```python
from build123d import *

# Parameters (mm, degrees)
SKETCH_1_W                    = 96
SKETCH_1_H                    = 47
EXTRUDE_1_DEPTH               = 6
FILLET_1_R                    = 1
HOLE_WIZARD_M10_1_D           = 8.5
HOLE_WIZARD_M10_1_CSINK_D     = 10.05
HOLE_WIZARD_M10_1_CSINK_ANGLE = 90
SKETCH_2_R                    = 3.3
CUT_EXTRUDE_1_DEPTH           = 10
FILLET_2_R                    = 0.5


with BuildPart() as part:
    # 草图1 → 凸台-拉伸1 (new body)
    with BuildSketch(Plane.XY):
        with Locations((48, -23.5)):
            Rectangle(SKETCH_1_W, SKETCH_1_H)
    extrude(amount=EXTRUDE_1_DEPTH)

    # 圆角1
    fillet_1_edges = [part.edges().sort_by_distance(p)[0] for p in [
        (0, 0, 3),
        (96, 0, 3),
        (96, -47, 3),
        (0, -47, 3),
    ]]
    fillet(fillet_1_edges, radius=FILLET_1_R)

    # M10 螺纹孔1 (through all)
    with Locations(Plane.XY.offset(6)):
        with Locations((28, -23.5), (48, -23.5), (68, -23.5)):
            CounterSinkHole(HOLE_WIZARD_M10_1_D / 2, HOLE_WIZARD_M10_1_CSINK_D / 2, counter_sink_angle=HOLE_WIZARD_M10_1_CSINK_ANGLE)

    # 草图2 → 切除-拉伸1 (cut)
    with BuildSketch(Plane.XY.offset(6)):
        with Locations((83, -6)):
            Circle(SKETCH_2_R)
        with Locations((83, -41)):
            Circle(SKETCH_2_R)
        with Locations((13, -41)):
            Circle(SKETCH_2_R)
        with Locations(Location((13, -6, 0), (0, 0, 180))):
            Circle(SKETCH_2_R)
    extrude(amount=-CUT_EXTRUDE_1_DEPTH, mode=Mode.SUBTRACT)

    # 圆角2
    fillet_2_edges = [part.edges().sort_by_distance(p)[0] for p in [
        (16.3, -6, 6),
        (9.7, -41, 6),
        (79.7, -41, 6),
        (79.7, -6, 6),
    ]]
    fillet(fillet_2_edges, radius=FILLET_2_R)


solid = part.part
```
The model under review builds one solid part; all positions refer to its coordinate system, in mm. Round coordinates to 2 decimals unless told otherwise and drop trailing zeros. Write each loop counter-clockwise with the first axis right and the second up, starting at its lowest first coordinate (ties: lowest second). Pieces come first, ordered by that corner, then holes. Notation, with made-up numbers: (34.25, -36.5) -> (38.25, -36.5) arc R20 ccw to (38.25, -30.5) -> close; hole circle Ø2 at (26, 22). An arc over 180 degrees is marked (long way). Use CSV: the item, a comma, the result in double quotes.
Q1. Consider section A-A (x = 13). Give the boundary of the cut face in (y, z).
Checks:
outline,"(-47, 0) -> (-44.3, 0) -> (-44.3, 5.5) arc R0.5 ccw to (-44.8, 6) -> (-47, 6) -> close; (-37.7, 0) -> (-9.3, 0) -> (-9.3, 5.5) arc R0.5 ccw to (-9.8, 6) -> (-37.2, 6) arc R0.5 ccw to (-37.7, 5.5) -> close; (-2.7, 0) -> (0, 0) -> (0, 6) -> (-2.2, 6) arc R0.5 ccw to (-2.7, 5.5) -> close"
Q2. Mouldability with a two-part tool opening along X and no side actions: class faces 1 (the flat face through (47, -18, 0)), 2 (the cylindrical face through (52.246, -23.313, 2.576)), 3 (the cylindrical face through (64.074, -25.128, 2.576)), 4 (the flat face through (0, -24, 3)) as released by +X, released by -X, zero draft, split by the parting line, or undercut.
Checks:
face 1,"zero draft"
face 2,"undercut"
face 3,"undercut"
face 4,"released by -X"
Q3. For pin 1 Ø7.5 at (x, y) = (83, -6) entering from -Z; pin 2 Ø10 at (x, y) = (68, -23.5) entering from +Z (3 decimals), all flat-tipped, find the tip position at first contact; note any pin that passes through.
Checks:
pin 1,"z = 0"
pin 2,"z = 5.975"
Q4. Consider section B-B (y = -6). Give the boundary of the cut face in (x, z).
Checks:
outline,"(0, 0) -> (9.7, 0) -> (9.7, 5.5) arc R0.5 ccw to (9.2, 6) -> (0, 6) -> close; (16.3, 0) -> (79.7, 0) -> (79.7, 5.5) arc R0.5 ccw to (79.2, 6) -> (16.8, 6) arc R0.5 ccw to (16.3, 5.5) -> close; (86.3, 0) -> (96, 0) -> (96, 6) -> (86.8, 6) arc R0.5 ccw to (86.3, 5.5) -> close"
Q5. To check wall thickness, follow probe 1 along X at (y, z) = (-23.5, 3.85); probe 2 along Y at (x, z) = (82, 2.5); probe 3 along Y at (x, z) = (28, 3.5). State the ranges of each line that lie inside material, in increasing order. Write a range as [from, to].
Checks:
probe 1,"[0, 23.75], [32.25, 43.75], [52.25, 63.75], [72.25, 96]"
probe 2,"[-47, -44.14], [-37.86, -9.14], [-2.86, 0]"
probe 3,"[-47, -27.75], [-19.25, 0]"
Q6. Consider section C-C (z = 2.5). Give the boundary of the cut face in (x, y), then the cut area to 3 significant figures.
Checks:
outline,"(0, -46) arc R1 ccw to (1, -47) -> (95, -47) arc R1 ccw to (96, -46) -> (96, -1) arc R1 ccw to (95, 0) -> (1, 0) arc R1 ccw to (0, -1) -> close; hole circle Ø6.6 at (13, -41); hole circle Ø6.6 at (13, -6); hole circle Ø8.5 at (28, -23.5); hole circle Ø8.5 at (48, -23.5); hole circle Ø8.5 at (68, -23.5); hole circle Ø6.6 at (83, -41); hole circle Ø6.6 at (83, -6)"
area,"4,200 mm²"
Q7. Consider section D-D (y = -23.5). Give the boundary of the cut face in (x, z) (3 decimals).
Checks:
outline,"(0, 0) -> (23.75, 0) -> (23.75, 5.225) -> (22.975, 6) -> (0, 6) -> close; (32.25, 0) -> (43.75, 0) -> (43.75, 5.225) -> (42.975, 6) -> (33.025, 6) -> (32.25, 5.225) -> close; (52.25, 0) -> (63.75, 0) -> (63.75, 5.225) -> (62.975, 6) -> (53.025, 6) -> (52.25, 5.225) -> close; (72.25, 0) -> (96, 0) -> (96, 6) -> (73.025, 6) -> (72.25, 5.225) -> close"
